Can you work these out from the drawing? Everything is in mm from the part's minimum corner. Coordinates: 2 decimals unless noted, no trailing zeros. Order: outer loops, then holes, each group sorted by start corner. A loop starts at its lowest first (then second) coordinate and runs counter-clockwise, first axis right, second up. Notation, with made-up numbers: (-38.5, 40.5) -> (2.5, 40.5) arc R4 cw to (2.5, 46.5) -> close; hole circle Ø7 at (13, 18). An arc over 180 degrees is marked (long way). Use a Markdown table: item, result. Add a question column.
1) Will this pin go through, and if not, where does the flat tip stop? pin 1 Ø1.5 at (x, z) = (68, 1) entering from -Y.
2) If we section it at B-B (x = 16): Write out the boundary of the cut face in (y, z), plus the area to 3 significant figures.
3) If I drill on L1, parallel to Y at x = 77, z = 1.2, over which ranges is the centre line in solid material (lowest first)? Write a range as [from, to].
4) If we section it at A-A (z = 0.95): Write out the boundary of the cut face in (x, y).
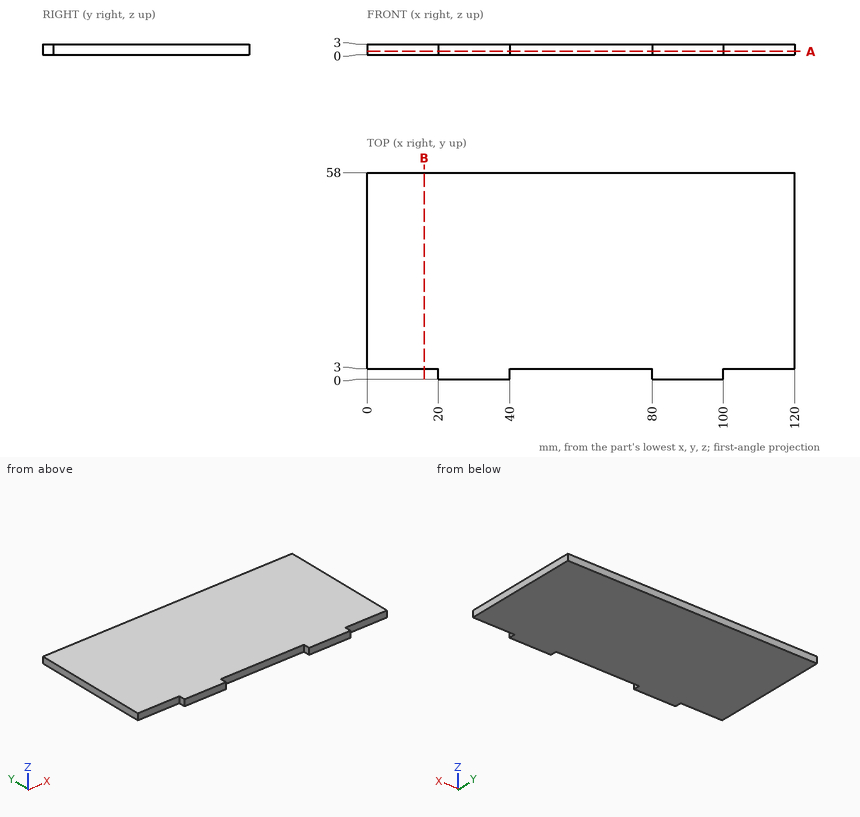
Answer sheet:
| question | item | result |
|---|---|---|
| 1 | pin 1 | y = 3 |
| 2 | outline | (3, 0) -> (58, 0) -> (58, 3) -> (3, 3) -> close |
| 2 | area | 165 mm2 |
| 3 | L1 | [3, 58] |
| 4 | outline | (0, 3) -> (20, 3) -> (20, 0) -> (40, 0) -> (40, 3) -> (80, 3) -> (80, 0) -> (100, 0) -> (100, 3) -> (120, 3) -> (120, 58) -> (0, 58) -> close |
